from build123d import *

# Parameters (mm, degrees)
F0_W     = 60
F0_H     = 70
F0_W_2   = 50
F0_H_2   = 60
F1_DEPTH = 60
F2_R     = 2
F3_R     = 3.5
F4_DEPTH = 35


with BuildPart() as f1:
    # F0 (on Top) → F1 (new body)
    with BuildSketch(Plane.XY):
        Rectangle(F0_W, F0_H)
        Rectangle(F0_W_2, F0_H_2, mode=Mode.SUBTRACT)
    extrude(amount=F1_DEPTH)

    # F2
    f2_edges = [f1.edges().sort_by_distance(p)[0] for p in [
        (-30, -35, 30),
        (30, -35, 30),
        (-30, 35, 30),
        (30, 35, 30),
        (25, -30, 30),
        (-25, 30, 30),
        (25, 30, 30),
        (-25, -30, 30),
    ]]
    fillet(f2_edges, radius=F2_R)

    # F3 (on Front) → F4 (cut, symmetric)
    with BuildSketch(Plane.XZ):
        with Locations((0, 10)):
            Circle(F3_R)
    extrude(amount=F4_DEPTH, both=True, mode=Mode.SUBTRACT)


solid = f1.part
Can you work these out from the model? Positions are in its coordinate system, mm. A direction names the side the tool comes from. Give positions to 0.01 mm unless a question says otherwise; leave off trailing zeros. Loops run counter-clockwise (first coordinate to the right, second up) from the corner with the lowest first, then second, coordinate; pieces in that order, holes last. Notation, with made-up numbers: (85.5, -21) - (136.5, -21) arc R27 cw to (136.5, 14) - close; hole circle Ø5 at (29, 51). An arc over 180 degrees is marked (long way). Return JSON: item names as keys, results as strings.
1. I want a section at B-B on y = -16. Please give me the cut outline in (x, z), and give its area (3 significant figures).
Output values:
{"outline": "(-30, 0) - (-25, 0) - (-25, 60) - (-30, 60) - close; (25, 0) - (30, 0) - (30, 60) - (25, 60) - close", "area": "600 mm²"}
2. I'm going to push a flat-ended pin straight in: pin 1 Ø8 at (x, z) = (0, 10) entering from -Y. Where does the tip first touch, or does it pass through?
Output values:
{"pin 1": "stops at y = -35"}
3. For faces 1 (the face through (-30, 0, 30)), 2 (the face through (0, -30, 30)), which set-ups out of +Z, -Z, +X, -X, +Y, -Y let a thin tool reach every point of the face, with its end or its side?
Output values:
{"face 1": "+Z, -Z, -X, +Y, -Y", "face 2": "+Z, -Z"}
4. If I drill on line 1 (Y direction, x = 4, z = 41); line 2 (X direction, y = -3, z = 13); line 3 (Z direction, x = 0, y = 32.2), over which ranges is the centre line in solid material (lowest first)?
Output values:
{"line 1": "y = -35 to -30, 30 to 35", "line 2": "x = -30 to -25, 25 to 30", "line 3": "z = 0 to 6.5, 13.5 to 60"}
5. We'd pull the mould along Z, two halves only. Please class faces 3 (the face through (0, -35, 30)), 4 (the face through (-0.759, -32.535, 6.583)), 5 (the face through (-0.759, 32.465, 6.583)), 6 (the face through (-27, 0, 0)): +Z half, -Z half, draft (parallel to the pull), parting line (faces both ways), or undercut.
Output values:
{"face 3": "draft", "face 4": "undercut", "face 5": "undercut", "face 6": "-Z half"}
6. I want a section at A-A on x = 0. Please give me the cut outline in (y, z), and give its area (3 significant figures).
Output values:
{"outline": "(-35, 0) - (-30, 0) - (-30, 6.5) - (-35, 6.5) - close; (-35, 13.5) - (-30, 13.5) - (-30, 60) - (-35, 60) - close; (30, 0) - (35, 0) - (35, 6.5) - (30, 6.5) - close; (30, 13.5) - (35, 13.5) - (35, 60) - (30, 60) - close", "area": "530 mm²"}
7. I want a section at C-C on z = 38. Please give me the cut outline in (x, y).
Output values:
{"outline": "(-30, -33) arc R2 ccw to (-28, -35) - (28, -35) arc R2 ccw to (30, -33) - (30, 33) arc R2 ccw to (28, 35) - (-28, 35) arc R2 ccw to (-30, 33) - close; hole (-25, -28) arc R2 ccw to (-23, -30) - (23, -30) arc R2 ccw to (25, -28) - (25, 28) arc R2 ccw to (23, 30) - (-23, 30) arc R2 ccw to (-25, 28) - close"}
8. I want a section at D-D on x = -8.5. Please give me the cut outline in (y, z), and give its area (3 significant figures).
Output values:
{"outline": "(-35, 0) - (-30, 0) - (-30, 60) - (-35, 60) - close; (30, 0) - (35, 0) - (35, 60) - (30, 60) - close", "area": "600 mm²"}
